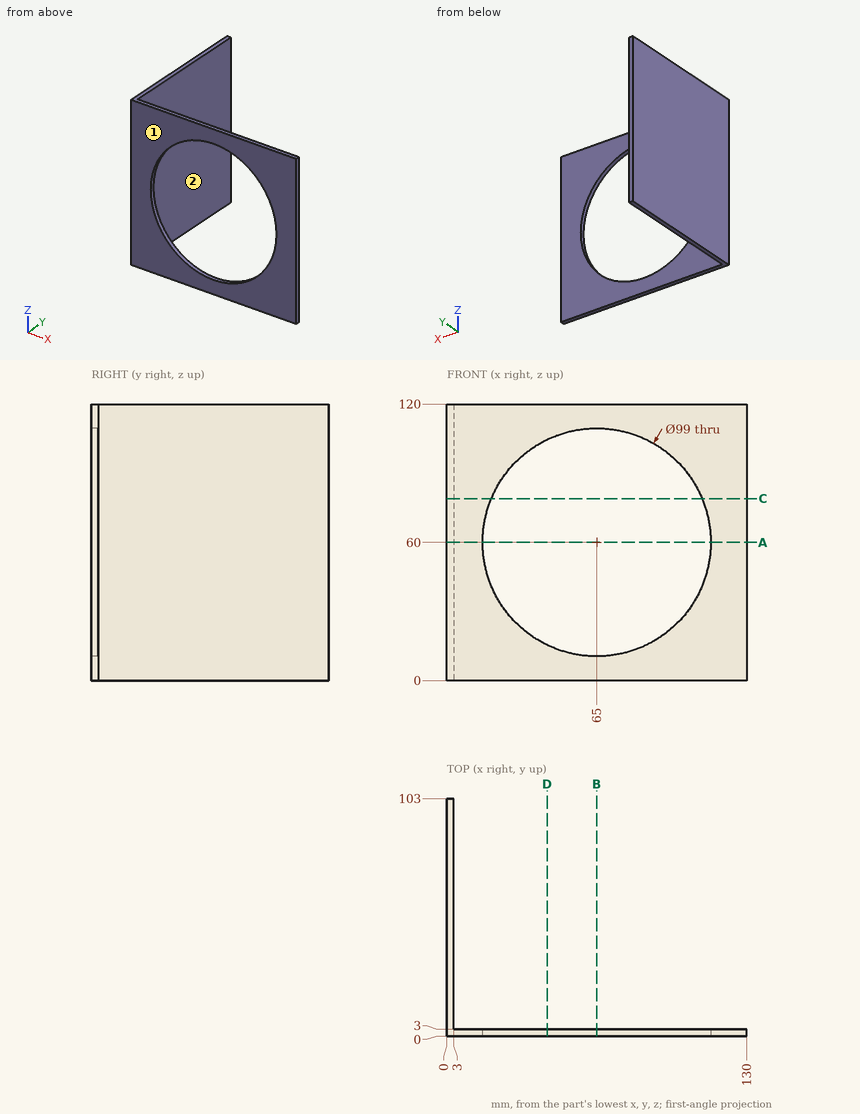
Answer from the drawing. Dimensions are ordinates in mm from the lowest x, y and z of the part. A direction names the side the tool comes from. Round coordinates to 2 decimals unless told otherwise and drop trailing zeros. Order: outer loops, then holes, each group sorted by start corner. A loop starts at its lowest first (then second) coordinate and runs counter-clockwise, first axis right, second up. Notation, with made-up numbers: (14, 22) -> (54, 22) arc R31 cw to (54, 50) -> close; hole circle Ø2 at (34, -11.5). An arc over 180 degrees is marked (long way). Answer as CSV lines item,"result".
Q1. Which of the six approach directions +Z, -Z, +X, -X, +Y, -Y give full straight-line access (tool end or side, diameter ignored) to the marked faces 1 and 2?
Computed values:
face 1,"+Z, -Z, +X, -X, -Y"
face 2,"+Z, -Z, +X, +Y"
Q2. A cutting plane is placed at B-B on x = 65. Determine the outline of the cut face in (y, z), plus the area to 3 significant figures.
Computed values:
outline,"(0, 0) -> (3, 0) -> (3, 10.5) -> (0, 10.5) -> close; (0, 109.5) -> (3, 109.5) -> (3, 120) -> (0, 120) -> close"
area,"63.0 mm^2"
Q3. A cutting plane is placed at D-D on x = 43.5. Determine the outline of the cut face in (y, z), plus the area to 3 significant figures.
Computed values:
outline,"(0, 0) -> (3, 0) -> (3, 15.41) -> (0, 15.41) -> close; (0, 104.59) -> (3, 104.59) -> (3, 120) -> (0, 120) -> close"
area,"92.5 mm^2"
Q4. A cutting plane is placed at C-C on z = 79. Determine the outline of the cut face in (x, y), plus the area to 3 significant figures.
Computed values:
outline,"(0, 0) -> (19.29, 0) -> (19.29, 3) -> (3, 3) -> (3, 103) -> (0, 103) -> close; (110.71, 0) -> (130, 0) -> (130, 3) -> (110.71, 3) -> close"
area,"416 mm^2"
Q5. Given pin 1 (3 mm diameter, centred on x = 14.5, z = 62.5, fed in from -Y), flat-ended and moving along its own axis, determine where the tip first touches the part or whether it passes through.
Computed values:
pin 1,"stops at y = 0"
Q6. A cutting plane is placed at A-A on z = 60. Determine the outline of the cut face in (x, y), plus the area to 3 significant figures.
Computed values:
outline,"(0, 0) -> (15.5, 0) -> (15.5, 3) -> (3, 3) -> (3, 103) -> (0, 103) -> close; (114.5, 0) -> (130, 0) -> (130, 3) -> (114.5, 3) -> close"
area,"393 mm^2"
Q7. Consider line 1 (Z direction, x = 65, y = 1.15); line 2 (X direction, y = 60.5, z = 112). Determine where each line is inside the solid, lowest interval first. Write a range as from..to.
Computed values:
line 1,"z = 0..10.5, 109.5..120"
line 2,"x = 0..3"
